Check sheet for the modelled part. Datum: model origin and axes. Units: mm. Face numbers are marked on the shaded views. Round coordinates to 2 decimals unless told otherwise and drop trailing zeros. Write each loop counter-clockwise with the first axis right and the second up, starting at its lowest first coordinate (ties: lowest second). Pieces come first, ordered by that corner, then holes. Notation, with made-up numbers: M 51.5,7.25 L 70.5,7.25 A12 ccw 70.5,25.25 Z; hole C 75,38 d8. An arc over 180 degrees is marked long. Put each result on its own line as item: value.
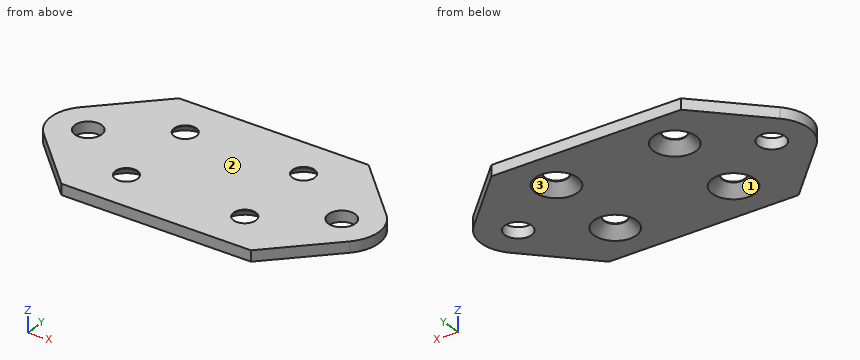
```python
from build123d import *

# Parameters (mm, degrees)
SKETCH1_R                                      = 4
BOSS_EXTRUDE1_DEPTH                            = 3.2
CSK_FOR_M6_FLAT_HEAD_MACHINE_SCREW1_AT_2_COUNT = 2
CSK_FOR_M6_FLAT_HEAD_MACHINE_SCREW1_AT_2_PITCH = 25
CSK_FOR_M6_FLAT_HEAD_MACHINE_SCREW1_AT_3_COUNT = 2
CSK_FOR_M6_FLAT_HEAD_MACHINE_SCREW1_AT_3_PITCH = 43.011626335
CSK_FOR_M6_FLAT_HEAD_MACHINE_SCREW1_AT_4_COUNT = 2
CSK_FOR_M6_FLAT_HEAD_MACHINE_SCREW1_AT_4_PITCH = 35


with BuildPart() as part:
    # Sketch1 → Boss-Extrude1 (new body)
    with BuildSketch(Plane.XY):
        with BuildLine():
            Line((9.443650814, 25), (65.556349186, 25))
            Line((65.556349186, 25), (82.778174593, 7.778174593))
            ThreePointArc((82.778174593, 7.778174593), (86, 0), (82.778174593, -7.778174593))
            Line((82.778174593, -7.778174593), (65.556349186, -25))
            Line((65.556349186, -25), (9.443650814, -25))
            Line((9.443650814, -25), (-7.778174593, -7.778174593))
            ThreePointArc((-7.778174593, -7.778174593), (-11, 0), (-7.778174593, 7.778174593))
            Line((-7.778174593, 7.778174593), (9.443650814, 25))
        make_face()
        Circle(SKETCH1_R, mode=Mode.SUBTRACT)
        with Locations((75, 0)):
            Circle(SKETCH1_R, mode=Mode.SUBTRACT)
    extrude(amount=BOSS_EXTRUDE1_DEPTH)

    # Sketch13 → CSK for M6 Flat Head Machine Screw1 (revolve, cut)
    with BuildSketch(Plane(origin=(20, -12.5, 0), x_dir=(0, 1, 0), z_dir=(1, 0, 0))):
        Polygon((0, 0), (0, 3.2), (3.3, 3.2), (3.3, 3), (6.3, 0), align=None)
    csk_for_m6_flat_head_machine_screw1 = revolve(axis=Axis((20, -12.5, -6.35), (0, 0, 1)), mode=Mode.SUBTRACT)

    # CSK for M6 Flat Head Machine Screw1 at 2: CSK for M6 Flat Head Machine Screw1 ×2
    with Locations(*[(0, i * CSK_FOR_M6_FLAT_HEAD_MACHINE_SCREW1_AT_2_PITCH, 0) for i in range(1, CSK_FOR_M6_FLAT_HEAD_MACHINE_SCREW1_AT_2_COUNT)]):
        add(csk_for_m6_flat_head_machine_screw1, mode=Mode.SUBTRACT)

    # CSK for M6 Flat Head Machine Screw1 at 3: CSK for M6 Flat Head Machine Screw1 ×2
    with Locations(*[Vector(0.813733471, 0.581238194, 0) * (i * CSK_FOR_M6_FLAT_HEAD_MACHINE_SCREW1_AT_3_PITCH) for i in range(1, CSK_FOR_M6_FLAT_HEAD_MACHINE_SCREW1_AT_3_COUNT)]):
        add(csk_for_m6_flat_head_machine_screw1, mode=Mode.SUBTRACT)

    # CSK for M6 Flat Head Machine Screw1 at 4: CSK for M6 Flat Head Machine Screw1 ×2
    with Locations(*[(i * CSK_FOR_M6_FLAT_HEAD_MACHINE_SCREW1_AT_4_PITCH, 0, 0) for i in range(1, CSK_FOR_M6_FLAT_HEAD_MACHINE_SCREW1_AT_4_COUNT)]):
        add(csk_for_m6_flat_head_machine_screw1, mode=Mode.SUBTRACT)


solid = part.part
```
1. Cross-section at B-B (z = 0.6). Enter the section's corners in (x, y), then the cut area to 3 significant figures.
Computed values:
outline: M -7.78,-7.78 L 9.44,-25 L 65.56,-25 L 82.78,-7.78 A11 ccw 82.78,7.78 L 65.56,25 L 9.44,25 L -7.78,7.78 A11 ccw Z; hole C 0,0 d8; hole C 20,-12.5 d11.4; hole C 20,12.5 d11.4; hole C 55,-12.5 d11.4; hole C 55,12.5 d11.4; hole C 75,0 d8
area: 3,490 mm2
2. Cross-section at C-C (y = -12.5). Enter the section's corners in (x, z), then the cut area to 3 significant figures.
Computed values:
outline: M -3.06,0 L 13.7,0 L 16.7,3 L 16.7,3.2 L -3.06,3.2 Z; M 23.3,3 L 26.3,0 L 48.7,0 L 51.7,3 L 51.7,3.2 L 23.3,3.2 Z; M 58.3,3 L 61.3,0 L 78.06,0 L 78.06,3.2 L 58.3,3.2 Z
area: 199 mm2
3. Cross-section at D-D (x = 0). Enter the section's corners in (y, z), then the cut area to 3 significant figures.
Computed values:
outline: M -15.56,0 L -4,0 L -4,3.2 L -15.56,3.2 Z; M 4,0 L 15.56,0 L 15.56,3.2 L 4,3.2 Z
area: 74.0 mm2
4. Release check for a two-part mould opening along X. For the marked faces 1, 2 and 3 record: +X half, -X half, draft (parallel to the pull), parting line (faces both ways), or undercut.
Computed values:
face 1: undercut
face 2: draft
face 3: undercut
5. Depth check by flat-ended pin: pin 1 Ø5.5 at (x, y) = (55, -12.5) entering from +Z; pin 2 Ø8.5 at (x, y) = (20, 12.5) entering from -Z. Enter the tip coordinate at first touch or a pass-through.
Computed values:
pin 1: passes through
pin 2: stops at z = 2.05
6. Cross-section at A-A (x = 55). Enter the section's corners in (y, z), then the cut area to 3 significant figures.
Computed values:
outline: M -25,0 L -18.8,0 L -15.8,3 L -15.8,3.2 L -25,3.2 Z; M -9.2,3 L -6.2,0 L 6.2,0 L 9.2,3 L 9.2,3.2 L -9.2,3.2 Z; M 15.8,3 L 18.8,0 L 25,0 L 25,3.2 L 15.8,3.2 Z
area: 99.8 mm2
7. Scan lines: probe 1 along Y at (x, z) = (20, 3.1); probe 2 along X at (y, z) = (-12.5, 3.15); probe 3 along X at (y, z) = (-9, 0.35). Record each from-to range of solid material in increasing order.
Computed values:
probe 1: y = -25 to -15.8, -9.2 to 9.2, 15.8 to 25
probe 2: x = -3.06 to 16.7, 23.3 to 51.7, 58.3 to 78.06
probe 3: x = -6.56 to 15.19, 24.81 to 50.19, 59.81 to 81.56
